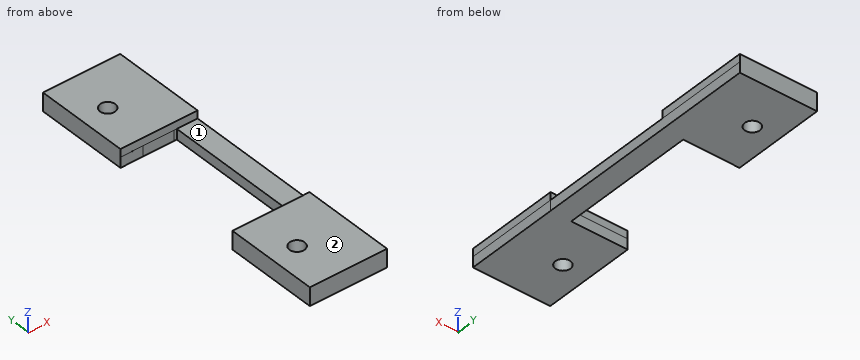
Autodesk Inventor part; units mm, degrees
ref_plane "YZ Plane" through (0, 0, 0) normal (1, 0, 0) x (0, 1, 0)
ref_plane "XZ Plane" through (0, 0, 0) normal (0, 1, 0) x (-1, 0, 0)
ref_plane "XY Plane" through (0, 0, 0) normal (0, 0, 1) x (1, 0, 0)
sketch "Sketch1" plane through (0, 0, 0) normal (0, 0, 1) x (1, 0, 0)
  circle A0 centre (14.9935, -706.254) radius 1.4499
  circle A1 centre (14.9932, -750.254) radius 1.4502
  line L0 (24.8521, -741.254) -> (24.8525, -697.2541)
  line L1 (24.8519, -759.254) -> (24.8521, -741.254)
  line L2 (20.3016, -715.254) -> (14.3016, -715.254)
  line L3 (9.9969, -697.2539) -> (24.8525, -697.2541)
  line L4 (24.8525, -697.2541) -> (24.8527, -715.2539)
  line L5 (24.8527, -715.2539) -> (24.8527, -715.2539)
  line L6 (24.8521, -741.254) -> (9.9968, -741.2539)
  line L7 (9.9968, -741.2539) -> (9.9968, -759.2539)
  line L8 (9.9968, -759.2539) -> (24.8519, -759.254)
  line L9 (24.8519, -759.254) -> (24.8521, -741.254)
  line L10 (24.8527, -715.2539) -> (9.9968, -715.2538)
  line L11 (9.9969, -697.2539) -> (9.9968, -715.2538)
  line L12 (24.8527, -715.2539) -> (24.8521, -741.254)
  line L13 (24.8521, -741.254) -> (20.8521, -741.254)
  line L14 (20.8521, -741.254) -> (20.8522, -715.2538)
  point P0 (0, 0)
  point P1 (24.8523, -715.2539)
extrude "Extrusion1" add sketch "Sketch1" along normal blind 2
sketch "Sketch3" plane through (0, 0, 2) normal (0, 0, 1) x (1, 0, 0)
  line L0 (9.9968, -715.2538) -> (20.8522, -715.2538)
  line L1 (20.8522, -715.2538) -> (20.8521, -741.254)
  line L2 (20.8521, -741.254) -> (9.9968, -741.2539)
  line L3 (9.9968, -741.2539) -> (9.9968, -759.2539)
  line L4 (9.9968, -759.2539) -> (24.8519, -759.254)
  line L5 (24.8519, -759.254) -> (24.8525, -697.2541)
  line L6 (24.8525, -697.2541) -> (9.9969, -697.2539)
  line L7 (9.9969, -697.2539) -> (9.9968, -715.2538)
  circle A0 centre (14.9935, -706.254) radius 1.4499
  circle A1 centre (14.9932, -750.254) radius 1.4502
  line L8 (9.9968, -715.2538) -> (20.8522, -715.2538)
  line L9 (20.8522, -715.2538) -> (24.8523, -715.2538)
  line L10 (24.8519, -759.254) -> (24.8525, -697.2541)
  line L11 (20.8522, -715.2538) -> (20.8521, -741.254)
  line L12 (20.8521, -741.254) -> (24.8521, -741.254)
  point P0 (0, 0)
extrude "Extrusion3" add sketch "Sketch3" along normal blind 1.5 contours L7 L6 L5 L9 L0 | L12 L5 L4 L3 L2
properties part number "imu_cable_holder"
CAD build for the part. Positions are in the model's coordinates, mm. Face numbers are marked on the shaded views. Give positions to 0.01 mm unless a question says otherwise; leave off trailing zeros. Loops run counter-clockwise (first coordinate to the right, second up) from the corner with the lowest first, then second, coordinate; pieces in that order, holes last. Notation, with made-up numbers: (30, -18) - (35, -18) arc R13 cw to (35, -13) - close; hole circle Ø8 at (73.5, 63). An arc over 180 degrees is marked (long way). Put each result on its own line as item: value.
Q1. Slice it at D-D (z = 0.6). Give the cut face in (x, y), plus the area to 3 significant figures.
Filled in:
outline: (10, -759.25) - (24.85, -759.25) - (24.85, -741.25) - (24.85, -697.25) - (10, -697.25) - (10, -715.25) - (14.3, -715.25) - (20.3, -715.25) - (20.85, -715.25) - (20.85, -741.25) - (10, -741.25) - close; hole circle Ø2.9 at (14.99, -750.25); hole circle Ø2.9 at (14.99, -706.25)
area: 626 mm²
Q2. Flat gauge pin, fed straight in: pin 1 (1.5 mm diameter, centred on y = -725, z = 2.5, fed in from -X). Where does the tip first touch, or does it go through?
Filled in:
pin 1: stops at x = 20.85
Q3. Mould opens along Y. For the marked faces 1 and 2 say: pulls with the +Y half, pulls with the -Y half, needs draft (parallel to the pull), parting line crosses it, or undercut.
Filled in:
face 1: undercut
face 2: needs draft
Q4. Slice it at A-A (z = 2.95). Give the cut face in (x, y), plus the area to 3 significant figures.
Filled in:
outline: (10, -759.25) - (24.85, -759.25) - (24.85, -741.25) - (20.85, -741.25) - (10, -741.25) - close; (10, -715.25) - (24.85, -715.25) - (24.85, -697.25) - (10, -697.25) - close; hole circle Ø2.9 at (14.99, -750.25); hole circle Ø2.9 at (14.99, -706.25)
area: 522 mm²
Q5. Probe line 1 along Y through (x, z) = (15.5, 1.4); line 2 along Y through (x, z) = (13.5, 1.9); line 3 along Y through (x, z) = (16, 2.45). List the from-to ranges inside material, lowest first.
Filled in:
line 1: y = -759.25 to -751.61, -748.9 to -741.25, -715.25 to -707.61, -704.9 to -697.25
line 2: y = -759.25 to -741.25, -715.25 to -697.25
line 3: y = -759.25 to -751.3, -749.21 to -741.25, -715.25 to -707.3, -705.21 to -697.25
Q6. Slice it at B-B (x = 15.25). Give the number of separate pieces and of enclosed holes in the cut face, plus the area to 3 significant figures.
Filled in:
separate pieces: 4
enclosed holes: 0
area: 106 mm²
